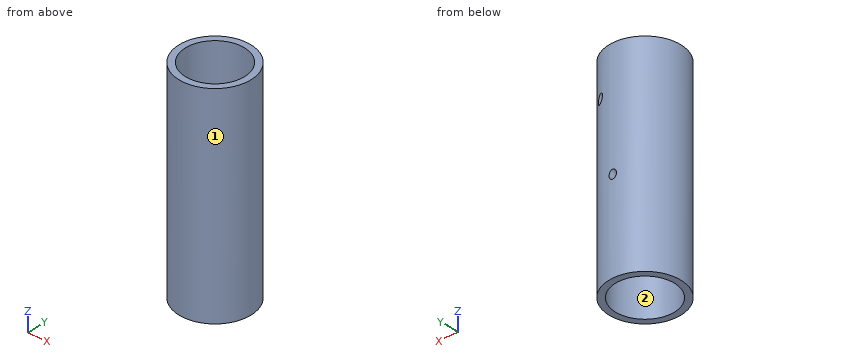
from build123d import *

# Parameters (mm, degrees)
SKIZZE1_R                       = 27.484712029
SKIZZE1_R_2                     = 22.58736277
AUFSATZ_LINEAR_AUSTRAGEN1_DEPTH = 160


with BuildPart() as part:
    # Skizze1 → Aufsatz-Linear austragen1 (new body)
    with BuildSketch(Plane.XY):
        Circle(SKIZZE1_R)
        Circle(SKIZZE1_R_2, mode=Mode.SUBTRACT)
    extrude(amount=-AUFSATZ_LINEAR_AUSTRAGEN1_DEPTH)

    # Skizze6 → Ø6.0 (6) Durchmesser Bohrung2 (revolve, cut)
    with BuildSketch(Plane(origin=(0, 0, -107.118504804), x_dir=(0, 0.544639035, -0.838670568), z_dir=(1, 0, 0))):
        Polygon((0, 0), (0, 83.113387119), (2.865, 81.391921446), (2.865, 0), align=None)
    revolve(axis=Axis((0, -5.325558106, -110.576962677), (0, 0.838670568, 0.544639035)), mode=Mode.SUBTRACT)

    # Skizze9 → Ø6.0 (6) Durchmesser Bohrung3 (revolve, cut)
    with BuildSketch(Plane(origin=(12, -1.983133308, -48.982393542), x_dir=(0, 0.544639035, -0.838670568), z_dir=(1, 0, 0))):
        Polygon((0, 0), (0, 53.059309664), (2.775, 51.391921446), (2.775, 0), align=None)
    revolve(axis=Axis((12, -7.308691414, -52.440851414), (0, 0.838670568, 0.544639035)), mode=Mode.SUBTRACT)


solid = part.part
The listing builds one solid part. Answer for the finished solid, in the listing's coordinates (mm). Face numbers are marked on the shaded views. Coordinates: 2 decimals unless noted, no trailing zeros. Write each loop counter-clockwise with the first axis right and the second up, starting at its lowest first coordinate (ties: lowest second). Pieces come first, ordered by that corner, then holes. Notation, with made-up numbers: (11.5, 72) - (44.5, 72) arc R28 cw to (44.5, 101) - close; hole circle Ø2 at (67.25, 45.5). An arc over 180 degrees is marked (long way). Put each result on its own line as item: value.
1. The part is cut by section A-A on y = 0. Give the vertices of the cut face in (x, z).
Answer sheet:
outline: (-27.48, -160) - (-22.59, -160) - (-22.59, 0) - (-27.48, 0) - close; (22.59, -160) - (27.48, -160) - (27.48, 0) - (22.59, 0) - close
2. The part is cut by section B-B on x = 17.5. Give the vertices of the cut face in (y, z).
Answer sheet:
outline: (-21.19, -160) - (-14.28, -160) - (-14.28, 0) - (-21.19, 0) - close; (14.28, -160) - (21.19, -160) - (21.19, 0) - (14.28, 0) - close
3. Determine the mould class of the marked faces 1 and 2 for opening direction Y: pulls with the +Y half, pulls with the -Y half, needs draft (parallel to the pull), parting line crosses it, or undercut.
Answer sheet:
face 1: parting line crosses it
face 2: undercut
4. Flat-ended cylindrical pins translate along their axes: pin 1 Ø2 at (x, z) = (-14, -140) entering from -Y; pin 2 Ø10 at (x, z) = (-3, -72.5) entering from +Y; pin 3 Ø1.5 at (y, z) = (-1, -136) entering from -X; pin 4 Ø10 at (y, z) = (7, -39) entering from +X. Find the tip coordinate at first contact, or state that the pin passes through.
Answer sheet:
pin 1: stops at y = -24.22
pin 2: stops at y = 27.48
pin 3: stops at x = -27.48
pin 4: stops at x = 27.41
5. The part is cut by section D-D on z = -56.5. Give the vertices of the cut face in (x, y).
Answer sheet:
outline: circle Ø54.97 at (0, 0); hole circle Ø45.17 at (0, 0)
6. The part is cut by section C-C on x = 0. Give the vertices of the cut face in (y, z).
Answer sheet:
outline: (-27.48, -160) - (-22.59, -160) - (-22.59, 0) - (-27.48, 0) - close; (22.59, -160) - (27.48, -160) - (27.48, -92.69) - (22.59, -95.87) - close; (22.59, -89.03) - (27.48, -85.85) - (27.48, 0) - (22.59, 0) - close
7. Find the intervals of material crossed by line 1 along Y through (x, z) = (0, -20); line 2 along X through (y, z) = (16.5, -123.5); line 3 along Y through (x, z) = (3, -11), in increasing order. Write a range as from..to.
Answer sheet:
line 1: y = -27.48..-22.59, 22.59..27.48
line 2: x = -21.98..-15.43, 15.43..21.98
line 3: y = -27.32..-22.39, 22.39..27.32
